CAD build for the part. Positions are in the model's coordinates, mm. A direction names the side the tool comes from. Give positions to 0.01 mm unless a question says otherwise; leave off trailing zeros. Loops run counter-clockwise (first coordinate to the right, second up) from the corner with the lowest first, then second, coordinate; pieces in that order, holes last.
Item 1: Mould opens along Y. For faces 1 (the flat face through (-31, 0, 3)), 2 (the flat face through (-158.3, 1.7, 3)), 3 (the flat face through (-79, 95, 3)) say: released by +Y, released by -Y, zero draft, split by the parting line, or undercut.
Item 2: Saw through at D-D on z = 4.75. Give the number of separate pieces and of enclosed holes in the cut face, plus the area to 3 significant figures.
Item 3: Saw through at B-B on y = 12.5. Give the cut face in (x, z).
Item 4: Probe probe 1 along X at (y, z) = (71, 1.5); probe 2 along X at (y, z) = (45.5, 2); probe 3 along X at (y, z) = (33.5, 1.95). List the from-to ranges inside material, lowest first.
Item 5: Drop flat-ended pins along their axis: P1, Ø5.5, axis at x = -273, y = 3, coming from the -Z side; P2, Ø1.5, axis at x = -209, z = 5, coming from the +Y side; P3, Ø1.5, axis at x = -133.5, z = 3, coming from the +Y side; P4, Ø2.5, axis at x = -133, z = 2.5, coming from the -Y side. Give the stop position or say it passes through.
Item 6: Which spindle directions (+Z, -Z, +X, -X, +Y, -Y) get a long thin tool onto all of the face, cutting with end or side? Do faces 4 (the cylindrical face through (-51.857, 3.9, 1.479)), 5 (the flat face through (-275, 89, 3)), 6 (the flat face through (-135, 44, 3)), 7 (the flat face through (-202, 79, 3)). Say none if no direction does.
Item 7: Saw through at A-A on y = 56.5. Give the cut face in (x, z).
Item 8: Saw through at C-C on x = -214. Give the cut face in (y, z), plus the area to 3 significant figures.
from build123d import *

# Parameters (mm, degrees)
ESQUISSE2_W             = 330
ESQUISSE2_H             = 95
BOSS_EXTRU_1_DEPTH      = 6
ESQUISSE3_W             = 6
ESQUISSE3_H             = 39
ESQUISSE3_W_2           = 60
ESQUISSE3_H_2           = 6
ESQUISSE3_H_3           = 30
ESQUISSE3_W_3           = 3
ENL_V_MAT_EXTRU_1_DEPTH = 344.45450936
ESQUISSE4_W             = 56.799161249
ESQUISSE4_H             = 89
ENL_V_MAT_EXTRU_2_DEPTH = 344.45450936
ESQUISSE5_R             = 1.5
ENL_V_MAT_EXTRU_3_DEPTH = 296.738059776
ESQUISSE6_R             = 2.995
ENL_V_MAT_EXTRU_5_DEPTH = 3


with BuildPart() as part:
    # Esquisse2 → Boss.-Extru.1 (new body)
    with BuildSketch(Plane.XY):
        with Locations((-165, 47.5)):
            Rectangle(ESQUISSE2_W, ESQUISSE2_H)
    extrude(amount=BOSS_EXTRU_1_DEPTH)

    # Esquisse3 → Enlèv. mat.-Extru.1 (cut, through all)
    with BuildSketch(Plane.XY.offset(6)):
        Polygon((-60, 95), (0, 95), (0, 59), (-6, 59), (-6, 89), (-20, 89), (-20, 69), (-60, 69), align=None)
        with Locations((-3, 19.5)):
            Rectangle(ESQUISSE3_W, ESQUISSE3_H)
        Polygon((-330, 95), (-270, 95), (-270, 89), (-324, 89), (-324, 59), (-330, 59), align=None)
        with Locations((-86, 3)):
            Rectangle(ESQUISSE3_W_2, ESQUISSE3_H_2)
        with Locations((-194, 3)):
            Rectangle(ESQUISSE3_W_2, ESQUISSE3_H_2)
        with Locations((-277, 44.5)):
            Rectangle(ESQUISSE3_W, ESQUISSE3_H_3)
        with Locations((-327, 19.5)):
            Rectangle(ESQUISSE3_W, ESQUISSE3_H)
        Polygon((-98, 95), (-98, 69), (-128, 69), (-128, 89), (-202, 89), (-202, 69), (-232, 69), (-232, 95), align=None)
        with Locations((-133.5, 44.5)):
            Rectangle(ESQUISSE3_W_3, ESQUISSE3_H_3)
    extrude(amount=-ENL_V_MAT_EXTRU_1_DEPTH, mode=Mode.SUBTRACT)

    # Esquisse4 → Enlèv. mat.-Extru.2 (cut, through all)
    with BuildSketch(Plane.XY.offset(6)):
        with Locations((-308.399580625, 44.5)):
            Rectangle(ESQUISSE4_W, ESQUISSE4_H)
    extrude(amount=-ENL_V_MAT_EXTRU_2_DEPTH, mode=Mode.SUBTRACT)

    # Esquisse5 → Enlèv. mat.-Extru.3 (cut, through all)
    with BuildSketch(Plane(origin=(0, 0, 0), x_dir=(-1, 0, 0), z_dir=(0, 0, -1))):
        with Locations((9, 3)):
            Circle(ESQUISSE5_R)
        with Locations((49, 3)):
            Circle(ESQUISSE5_R)
        with Locations((123, 3)):
            Circle(ESQUISSE5_R)
        with Locations((157, 3)):
            Circle(ESQUISSE5_R)
        with Locations((231, 3)):
            Circle(ESQUISSE5_R)
        with Locations((273, 3)):
            Circle(ESQUISSE5_R)
    extrude(amount=-ENL_V_MAT_EXTRU_3_DEPTH, mode=Mode.SUBTRACT)

    # Esquisse6 → Enlèv. mat.-Extru.5 (cut)
    with BuildSketch(Plane(origin=(0, 0, 0), x_dir=(-1, 0, 0), z_dir=(0, 0, -1))):
        with Locations((9, 3)):
            Circle(ESQUISSE6_R)
        with Locations((49, 3)):
            Circle(ESQUISSE6_R)
        with Locations((123, 3)):
            Circle(ESQUISSE6_R)
        with Locations((157, 3)):
            Circle(ESQUISSE6_R)
        with Locations((273, 3)):
            Circle(ESQUISSE6_R)
        with Locations((231, 3)):
            Circle(ESQUISSE6_R)
    extrude(amount=-ENL_V_MAT_EXTRU_5_DEPTH, mode=Mode.SUBTRACT)


solid = part.part
Results below:
1. face 1: released by -Y
1. face 2: undercut
1. face 3: released by +Y
2. separate pieces: 1
2. enclosed holes: 7
2. area: 21,900 mm2
3. outline: (-280, 0) - (-6, 0) - (-6, 6) - (-280, 6) - close
4. probe 1: x = -280 to -232, -202 to -128, -98 to -60, -20 to -6
4. probe 2: x = -274 to -135, -132 to 0
4. probe 3: x = -274 to -135, -132 to -6
5. P1: stops at z = 3
5. P2: stops at y = 69
5. P3: stops at y = 89
5. P4: stops at y = 0
6. face 4: -Z
6. face 5: +Z, -Z, -X, +Y
6. face 6: +Z, -Z
6. face 7: +Z, -Z, +Y
7. outline: (-274, 0) - (-135, 0) - (-135, 6) - (-274, 6) - close; (-132, 0) - (0, 0) - (0, 6) - (-132, 6) - close
8. outline: (6, 0) - (69, 0) - (69, 6) - (6, 6) - close
8. area: 378 mm2
